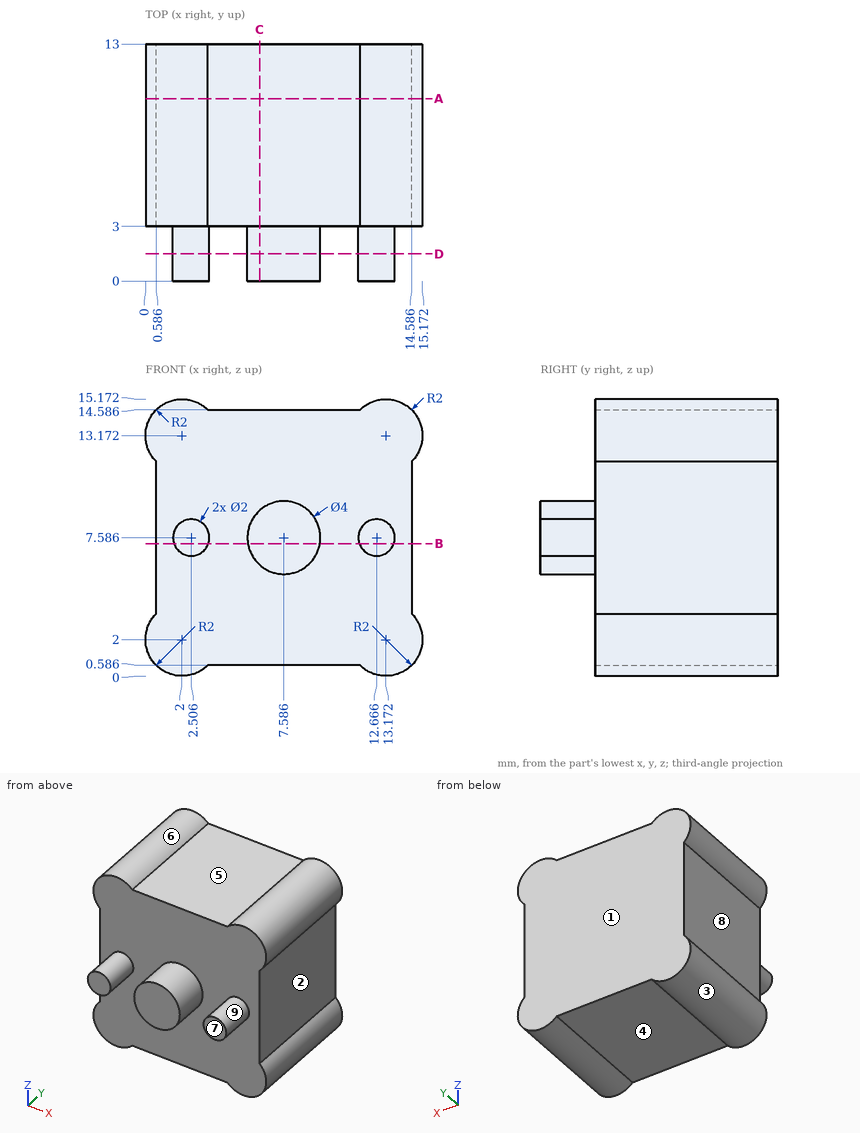
Job drawing, mm, ordinate dimensions from the low corner. One solid piece. A direction names the side the tool comes from. Give positions to 0.01 mm unless a question says otherwise; leave off trailing zeros. Order: outer loops, then holes, each group sorted by start corner. A loop starts at its lowest first (then second) coordinate and runs counter-clockwise, first axis right, second up. Notation, with made-up numbers: M -5.75,-20.75 L 53.25,-20.75 A18 cw 53.25,0.25 Z; hole C 51,26 d10. An arc over 180 degrees is marked long. Return JSON: item names as keys, results as strings.
Q1. Band-saw the part on C-C (x = 6.25). Give the cut face in (y, z) (1 decimal).
Answer list:
{"outline": "M 0,6.1 L 3,6.1 L 3,0.6 L 13,0.6 L 13,14.6 L 3,14.6 L 3,9.1 L 0,9.1 Z"}
Q2. 3-axis set-ups, long thin cutter, end or side, ignore diameter. For the marked faces 5, 6, 7, 8 and 9: which of +Z, -Z, +X, -X, +Y, -Y reach the whole face in a straight line?
Answer list:
{"face 5": "+Z, +Y, -Y", "face 6": "+Y, -Y", "face 7": "+Z, -Z, +X, -X, -Y", "face 8": "-X, +Y, -Y", "face 9": "-Y"}
Q3. Wall check: probe 1 along X at (y, z) = (1, 8) (1 decimal); probe 2 along Y at (x, z) = (1.5, 4.75); probe 3 along Z at (x, y) = (6.25, 4) (1 decimal). Give the ranges that are in metal, low to high. Write a range as from..to.
Answer list:
{"probe 1": "x = 1.6..3.4, 5.6..9.5, 11.8..13.6", "probe 2": "y = 3..13", "probe 3": "z = 0.6..14.6"}
Q4. Band-saw the part on B-B (z = 7.25). Give the cut face in (x, y) (1 decimal).
Answer list:
{"outline": "M 0.6,3 L 1.6,3 L 1.6,0 L 3.4,0 L 3.4,3 L 5.6,3 L 5.6,0 L 9.6,0 L 9.6,3 L 11.7,3 L 11.7,0 L 13.6,0 L 13.6,3 L 14.6,3 L 14.6,13 L 0.6,13 Z"}
Q5. Band-saw the part on D-D (y = 1.5). Give the cut face in (x, z) (1 decimal).
Answer list:
{"outline": "C 2.5,7.6 d2; C 7.6,7.6 d4; C 12.7,7.6 d2"}
Q6. Two-plate mould, pull along X, no slides. Class the marked faces 1, 2, 3 and 4: pulls with the +X half, pulls with the -X half, needs draft (parallel to the pull), parting line crosses it, or undercut.
Answer list:
{"face 1": "needs draft", "face 2": "pulls with the +X half", "face 3": "undercut", "face 4": "undercut"}
Q7. Band-saw the part on A-A (y = 10). Give the cut face in (x, z) (1 decimal).
Answer list:
{"outline": "M 0.6,3.4 A2 ccw 3.4,0.6 L 11.8,0.6 A2 ccw 14.6,3.4 L 14.6,11.8 A2 ccw 11.8,14.6 L 3.4,14.6 A2 ccw 0.6,11.8 Z"}
Q8. Flat gauge pins, fed straight in: pin 1 (2.5 mm diameter, centred on y = 9, z = 8.5, fed in from -X); pin 2 (2 mm diameter, centred on y = 9, z = 3.5, fed in from +X); pin 3 (6.5 mm diameter, centred on x = 5.5, y = 9, fed in from +Z). Where does each tip first touch, or does it go through?
Answer list:
{"pin 1": "stops at x = 0.59", "pin 2": "stops at x = 15.11", "pin 3": "stops at z = 15.16"}
